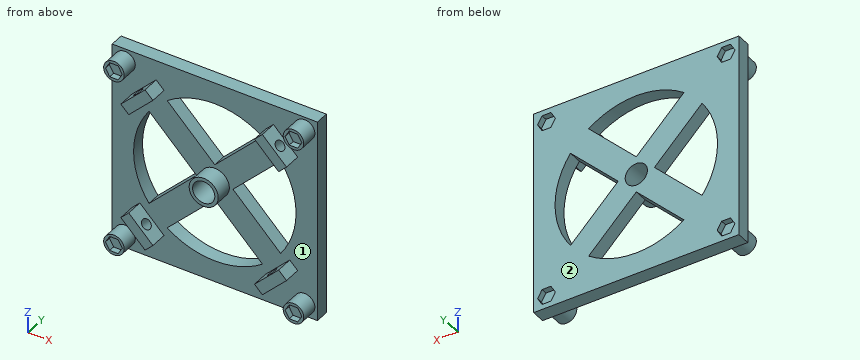
```python
from build123d import *

# Parameters (mm, degrees)
SKETCH2_W            = 120
SKETCH2_H            = 120
BOSS_EXTRUDE1_DEPTH  = 8
CUT_EXTRUDE1_DEPTH   = 3.5
LPATTERN1_COUNT      = 2
LPATTERN1_PITCH      = 105
LPATTERN1_COUNT_DIR2 = 2
LPATTERN1_PITCH_DIR2 = 105
AIR_HOLES_REACH      = 10
HEATER_MOUNTS_DEPTH  = 10
SKETCH14_R           = 3
HEATER_HOLES_DEPTH   = 6.5
CIRPATTERN2_COUNT    = 4
SKETCH11_R           = 8.5
BOSS_EXTRUDE3_DEPTH  = 10
CUT_EXTRUDE9_REACH   = 20
SKETCH16_R           = 6.5
SKETCH17_R           = 6
BOSS_EXTRUDE4_DEPTH  = 10
CUT_EXTRUDE10_DEPTH  = 3.5
LPATTERN4_COUNT      = 2
LPATTERN4_PITCH      = 105
LPATTERN4_COUNT_DIR2 = 2
LPATTERN4_PITCH_DIR2 = 105


with BuildPart() as part:
    # Sketch2 → Boss-Extrude1 (new body)
    with BuildSketch(Plane(origin=(0, 0, 0), x_dir=(1, 0, 0), z_dir=(0, 1, 0))):
        with Locations((-60, -60)):
            Rectangle(SKETCH2_W, SKETCH2_H)
    extrude(amount=BOSS_EXTRUDE1_DEPTH)

    # Sketch3 → Cut-Extrude1 (cut)
    with BuildSketch(Plane(origin=(0, 8, 0), x_dir=(1, 0, 0), z_dir=(0, 1, 0))):
        Polygon((-2.303847577, -112.5), (-4.901923789, -108), (-10.098076211, -108), (-12.696152423, -112.5), (-10.098076211, -117), (-4.901923789, -117), align=None)
    cut_extrude1 = extrude(amount=-CUT_EXTRUDE1_DEPTH, mode=Mode.SUBTRACT)

    # LPattern1: Cut-Extrude1 2 × 2
    with Locations(*[(-i * LPATTERN1_PITCH, 0, -j * LPATTERN1_PITCH_DIR2) for i in range(LPATTERN1_COUNT) for j in range(LPATTERN1_COUNT_DIR2) if (i, j) != (0, 0)]):
        add(cut_extrude1, mode=Mode.SUBTRACT)

    # Sketch8 → air holes (cut, up to next)
    with BuildSketch(Plane.XZ, mode=Mode.PRIVATE) as air_holes_sk1:
        with BuildLine():
            Line((-49.393398282, 60), (-21.530451238, 87.862947045))
            ThreePointArc((-21.530451238, 87.862947045), (-12.5, 60), (-21.530451238, 32.137052955))
            Line((-21.530451238, 32.137052955), (-49.393398282, 60))
        make_face()
    air_holes_tool1 = extrude(air_holes_sk1.sketch, amount=-AIR_HOLES_REACH, mode=Mode.PRIVATE) & part.part
    add(air_holes_tool1.solids().sort_by_distance((-26.860216, 0, 60))[0], mode=Mode.SUBTRACT)
    # Sketch8 → air holes (cut, up to next)
    with BuildSketch(Plane.XZ, mode=Mode.PRIVATE) as air_holes_sk2:
        with BuildLine():
            Line((-32.137052955, 21.530451238), (-60, 49.393398282))
            Line((-60, 49.393398282), (-87.862947045, 21.530451238))
            ThreePointArc((-87.862947045, 21.530451238), (-60, 12.5), (-32.137052955, 21.530451238))
        make_face()
    air_holes_tool2 = extrude(air_holes_sk2.sketch, amount=-AIR_HOLES_REACH, mode=Mode.PRIVATE) & part.part
    add(air_holes_tool2.solids().sort_by_distance((-60, 0, 26.860216))[0], mode=Mode.SUBTRACT)
    # Sketch8 → air holes (cut, up to next)
    with BuildSketch(Plane.XZ, mode=Mode.PRIVATE) as air_holes_sk3:
        with BuildLine():
            Line((-98.469548762, 32.137052955), (-70.606601718, 60))
            Line((-70.606601718, 60), (-98.469548762, 87.862947045))
            ThreePointArc((-98.469548762, 87.862947045), (-107.5, 60), (-98.469548762, 32.137052955))
        make_face()
    air_holes_tool3 = extrude(air_holes_sk3.sketch, amount=-AIR_HOLES_REACH, mode=Mode.PRIVATE) & part.part
    add(air_holes_tool3.solids().sort_by_distance((-93.139784, 0, 60))[0], mode=Mode.SUBTRACT)
    # Sketch8 → air holes (cut, up to next)
    with BuildSketch(Plane.XZ, mode=Mode.PRIVATE) as air_holes_sk4:
        with BuildLine():
            Line((-60, 70.606601718), (-32.137052955, 98.469548762))
            ThreePointArc((-32.137052955, 98.469548762), (-60, 107.5), (-87.862947045, 98.469548762))
            Line((-87.862947045, 98.469548762), (-60, 70.606601718))
        make_face()
    air_holes_tool4 = extrude(air_holes_sk4.sketch, amount=-AIR_HOLES_REACH, mode=Mode.PRIVATE) & part.part
    add(air_holes_tool4.solids().sort_by_distance((-60, 0, 93.139784))[0], mode=Mode.SUBTRACT)

    # Sketch13 → heater_mounts (add)
    with BuildSketch(Plane.XZ):
        Polygon((-16.159379566, 30.30151519), (-11.563185489, 25.705321112), (-25.705321112, 11.563185489), (-30.30151519, 16.159379566), align=None)
    heater_mounts = extrude(amount=HEATER_MOUNTS_DEPTH)

    # Sketch14 → heater_holes (cut)
    with BuildSketch(Plane(origin=(-23.230447378, 0, 23.230447378), x_dir=(0.707106781, 0, 0.707106781), z_dir=(-0.707106781, 0, 0.707106781))):
        with Locations((0, -5)):
            Circle(SKETCH14_R)
    heater_holes = extrude(amount=-HEATER_HOLES_DEPTH, mode=Mode.SUBTRACT)

    # CirPattern2: heater_mounts, heater_holes ×4 about axis
    cirpattern2_axis = Axis((-60, 0, 60), (0, 1, 0))
    for i in range(1, CIRPATTERN2_COUNT):
        add(heater_mounts.rotate(cirpattern2_axis, i * 360 / CIRPATTERN2_COUNT))
        add(heater_holes.rotate(cirpattern2_axis, i * 360 / CIRPATTERN2_COUNT), mode=Mode.SUBTRACT)

    # Sketch11 → Boss-Extrude3 (add)
    with BuildSketch(Plane.XZ):
        with Locations((-60, 60)):
            Circle(SKETCH11_R)
    extrude(amount=BOSS_EXTRUDE3_DEPTH)

    # Sketch16 → Cut-Extrude9 (cut, up to next)
    with BuildSketch(Plane.XZ.offset(10), mode=Mode.PRIVATE) as cut_extrude9_sk1:
        with Locations((-60, 60)):
            Circle(SKETCH16_R)
    cut_extrude9_tool1 = extrude(cut_extrude9_sk1.sketch, amount=-CUT_EXTRUDE9_REACH, mode=Mode.PRIVATE) & part.part
    add(cut_extrude9_tool1.solids().sort_by_distance((-60, -10, 60))[0], mode=Mode.SUBTRACT)

    # Sketch17 → Boss-Extrude4 (add)
    with BuildSketch(Plane.XZ):
        with Locations((-112.5, 112.5)):
            Circle(SKETCH17_R)
    boss_extrude4 = extrude(amount=BOSS_EXTRUDE4_DEPTH)

    # Sketch18 → Cut-Extrude10 (cut)
    with BuildSketch(Plane.XZ.offset(10)):
        Polygon((-117.407477288, 112.5), (-114.953738644, 108.25), (-110.046261356, 108.25), (-107.592522712, 112.5), (-110.046261356, 116.75), (-114.953738644, 116.75), align=None)
    cut_extrude10 = extrude(amount=-CUT_EXTRUDE10_DEPTH, mode=Mode.SUBTRACT)

    # LPattern4: Boss-Extrude4, Cut-Extrude10 2 × 2
    with Locations(*[(i * LPATTERN4_PITCH, 0, -j * LPATTERN4_PITCH_DIR2) for i in range(LPATTERN4_COUNT) for j in range(LPATTERN4_COUNT_DIR2) if (i, j) != (0, 0)]):
        add(boss_extrude4)
        add(cut_extrude10, mode=Mode.SUBTRACT)


solid = part.part
```
Check sheet for the modelled part. Datum: model origin and axes. Units: mm. Face numbers are marked on the shaded views. Round coordinates to 2 decimals unless told otherwise and drop trailing zeros. Order: outer loops, then holes, each group sorted by start corner. A loop starts at its lowest first (then second) coordinate and runs counter-clockwise, first axis right, second up.
1) Go/stop test with flat-tipped pins: pin 1 Ø1 at (y, z) = (5, 19.5) entering from +X; pin 2 Ø1.8 at (x, y) = (-7.5, -7.5) entering from +Z; pin 3 Ø1 at (x, y) = (-7.5, -8) entering from -Z; pin 4 Ø4 at (x, z) = (-8.5, 114.5) entering from -Y. Record where each tip stops, or that it passes through.
2) Section check A-A (z = 78). Record the boundary of the cut face in (x, y).
3) Section check B-B (x = -112.5). Record the boundary of the cut face in (y, z).
4) Mould release check, pull along Z, two halves, no side actions. Record for the marked faces 1 and 2: +Z half, -Z half, draft (parallel to the pull), parting line (faces both ways), or undercut.
5) Section check D-D (z = 63). Record the boundary of the cut face in (x, y).
6) Section check C-C (x = -84.5). Record the boundary of the cut face in (y, z).
7) Scan lines: line 1 (Z direction, x = -7.5, y = 4.75); line 2 (Z direction, x = -60, y = -3.5); line 3 (X direction, y = -5.5, z = 112). Record each from-to range of solid material in increasing order.
Result:
1. pin 1: stops at x = 0
1. pin 2: stops at z = 118.5
1. pin 3: stops at z = 1.5
1. pin 4: stops at y = -6.5
2. outline: (-120, 0) - (-103.96, 0) - (-103.96, 8) - (-120, 8) - close; (-88.61, 0) - (-67.39, 0) - (-67.39, 8) - (-88.61, 8) - close; (-52.61, 0) - (-31.39, 0) - (-31.39, 8) - (-52.61, 8) - close; (-16.04, 0) - (0, 0) - (0, 8) - (-16.04, 8) - close
3. outline: (-10, 1.5) - (0, 1.5) - (0, 0) - (8, 0) - (8, 3) - (4.5, 3) - (4.5, 12) - (8, 12) - (8, 108) - (4.5, 108) - (4.5, 117) - (8, 117) - (8, 120) - (0, 120) - (0, 118.5) - (-10, 118.5) - (-10, 116.75) - (-6.5, 116.75) - (-6.5, 108.25) - (-10, 108.25) - (-10, 106.5) - (0, 106.5) - (0, 13.5) - (-10, 13.5) - (-10, 11.75) - (-6.5, 11.75) - (-6.5, 3.25) - (-10, 3.25) - close
4. face 1: undercut
4. face 2: draft
5. outline: (-120, 0) - (-107.41, 0) - (-107.41, 8) - (-120, 8) - close; (-73.61, 0) - (-67.95, 0) - (-67.95, -10) - (-65.77, -10) - (-65.77, 8) - (-73.61, 8) - close; (-54.23, -10) - (-52.05, -10) - (-52.05, 0) - (-46.39, 0) - (-46.39, 8) - (-54.23, 8) - close; (-12.59, 0) - (0, 0) - (0, 8) - (-12.59, 8) - close
6. outline: (0, 0) - (8, 0) - (8, 19.31) - (0, 19.31) - close; (0, 24.89) - (8, 24.89) - (8, 46.11) - (0, 46.11) - close; (0, 73.89) - (8, 73.89) - (8, 95.11) - (0, 95.11) - close; (0, 100.69) - (8, 100.69) - (8, 120) - (0, 120) - close
7. line 1: z = 0 to 3, 12 to 108, 117 to 120
7. line 2: z = 51.5 to 53.5, 66.5 to 68.5
7. line 3: x = -118.48 to -106.52, -13.48 to -1.52
